```python
from build123d import *

# Parameters (mm, degrees)
EXTRUDE1_DEPTH                  = 75
F_1_2_0_500000_DIAMETER_HOLE1_D = 12.7
M6X1_0_TAPPED_HOLE1_D           = 6
LPATTERN1_COUNT                 = 2
LPATTERN1_PITCH                 = 25
LPATTERN1_COUNT_DIR2            = 2
LPATTERN1_PITCH_DIR2            = 25
M6X1_0_TAPPED_HOLE2_D           = 6
MIRROR2_COPY_1_D                = 6
MIRROR2_COPY_2_D                = 6
MIRROR2_COPY_3_D                = 6
MIRROR2_COPY_4_D                = 6
MIRROR3_COPY_1_D                = 6
MIRROR3_COPY_2_D                = 6
MIRROR3_COPY_3_D                = 6
MIRROR3_COPY_4_D                = 6
MIRROR3_COPY_5_D                = 6
MIRROR3_COPY_6_D                = 6
MIRROR3_COPY_7_D                = 6
MIRROR3_COPY_8_D                = 6
MIRROR3_COPY_9_D                = 6
MIRROR3_COPY_10_D               = 6


with BuildPart() as part:
    # Sketch1 → Extrude1 (new, symmetric)
    with BuildSketch(Plane.XY):
        Polygon((-67.79, 0), (67.79, 0), (67.79, 12.446), (75, 12.446), (75, 13.716), (-75, 13.716), (-75, 12.446), (-67.79, 12.446), align=None)
    extrude(amount=EXTRUDE1_DEPTH, both=True)

    # 1/2 (0.500000) Diameter Hole1 (through all)
    with Locations(Plane(origin=(0, 13.716, 0), x_dir=(-1, 0, 0), z_dir=(0, 1, 0))):
        with Locations((37.5, 25), (-37.5, 25), (-37.5, -25), (37.5, -25)):
            Hole(F_1_2_0_500000_DIAMETER_HOLE1_D / 2)

    # M6x1.0 Tapped Hole1 (through all)
    with Locations(Plane(origin=(0, 13.716, 0), x_dir=(-1, 0, 0), z_dir=(0, 1, 0))):
        with Locations((0, 0)):
            m6x1_0_tapped_hole1 = Hole(M6X1_0_TAPPED_HOLE1_D / 2)

    # LPattern1: M6x1.0 Tapped Hole1 2 × 2
    with Locations(*[(-i * LPATTERN1_PITCH, 0, -j * LPATTERN1_PITCH_DIR2) for i in range(LPATTERN1_COUNT) for j in range(LPATTERN1_COUNT_DIR2) if (i, j) != (0, 0)]):
        add(m6x1_0_tapped_hole1, mode=Mode.SUBTRACT)

    # M6x1.0 Tapped Hole2 (through all)
    with Locations(Plane(origin=(0, 13.716, 0), x_dir=(-1, 0, 0), z_dir=(0, 1, 0))):
        with Locations((37.5, -37.5), (50, -37.5), (50, -50)):
            m6x1_0_tapped_hole2 = Hole(M6X1_0_TAPPED_HOLE2_D / 2)

    # Mirror2: M6x1.0 Tapped Hole2 across plane
    add(m6x1_0_tapped_hole2.mirror(Plane.XY), mode=Mode.SUBTRACT)

    # Mirror2 copy 1 (through all)
    with Locations(Plane(origin=(0, 13.716, 25), x_dir=(-1, 0, 0), z_dir=(0, 1, 0))):
        with Locations((0, 0)):
            Hole(MIRROR2_COPY_1_D / 2)

    # Mirror2 copy 2 (through all)
    with Locations(Plane(origin=(-25, 13.716, 0), x_dir=(-1, 0, 0), z_dir=(0, 1, 0))):
        with Locations((0, 0)):
            Hole(MIRROR2_COPY_2_D / 2)

    # Mirror2 copy 3 (through all)
    with Locations(Plane(origin=(-25, 13.716, 25), x_dir=(-1, 0, 0), z_dir=(0, 1, 0))):
        with Locations((0, 0)):
            Hole(MIRROR2_COPY_3_D / 2)

    # Mirror2 copy 4 (through all)
    with Locations(Plane(origin=(0, 13.716, 0), x_dir=(-1, 0, 0), z_dir=(0, 1, 0))):
        with Locations((0, 0)):
            Hole(MIRROR2_COPY_4_D / 2)

    # Mirror3: M6x1.0 Tapped Hole2 across plane
    add(m6x1_0_tapped_hole2.mirror(Plane(origin=(0, 0, 0), x_dir=(0, 0, 1), z_dir=(1, 0, 0))), mode=Mode.SUBTRACT)

    # Mirror3 copy 1 (through all)
    with Locations(Plane(origin=(0, 13.716, -25), x_dir=(1, 0, 0), z_dir=(0, 1, 0))):
        with Locations((0, 0)):
            Hole(MIRROR3_COPY_1_D / 2)

    # Mirror3 copy 2 (through all)
    with Locations(Plane(origin=(25, 13.716, 0), x_dir=(1, 0, 0), z_dir=(0, 1, 0))):
        with Locations((0, 0)):
            Hole(MIRROR3_COPY_2_D / 2)

    # Mirror3 copy 3 (through all)
    with Locations(Plane(origin=(25, 13.716, -25), x_dir=(1, 0, 0), z_dir=(0, 1, 0))):
        with Locations((0, 0)):
            Hole(MIRROR3_COPY_3_D / 2)

    # Mirror3 copy 4 (through all)
    with Locations(Plane(origin=(0, 13.716, 0), x_dir=(1, 0, 0), z_dir=(0, 1, 0))):
        with Locations((0, 0)):
            Hole(MIRROR3_COPY_4_D / 2)

    # Mirror3 copy 5 (through all)
    with Locations(Plane(origin=(0, 13.716, 0), x_dir=(1, 0, 0), z_dir=(0, 1, 0))):
        with Locations((37.5, -37.5), (50, -37.5), (50, -50)):
            Hole(MIRROR3_COPY_5_D / 2)

    # Mirror3 copy 6 (through all)
    with Locations(Plane(origin=(0, 13.716, 25), x_dir=(1, 0, 0), z_dir=(0, 1, 0))):
        with Locations((0, 0)):
            Hole(MIRROR3_COPY_6_D / 2)

    # Mirror3 copy 7 (through all)
    with Locations(Plane(origin=(25, 13.716, 0), x_dir=(1, 0, 0), z_dir=(0, 1, 0))):
        with Locations((0, 0)):
            Hole(MIRROR3_COPY_7_D / 2)

    # Mirror3 copy 8 (through all)
    with Locations(Plane(origin=(25, 13.716, 25), x_dir=(1, 0, 0), z_dir=(0, 1, 0))):
        with Locations((0, 0)):
            Hole(MIRROR3_COPY_8_D / 2)

    # Mirror3 copy 9 (through all)
    with Locations(Plane(origin=(0, 13.716, 0), x_dir=(1, 0, 0), z_dir=(0, 1, 0))):
        with Locations((0, 0)):
            Hole(MIRROR3_COPY_9_D / 2)

    # Mirror3 copy 10 (through all)
    with Locations(Plane(origin=(0, 13.716, 0), x_dir=(1, 0, 0), z_dir=(0, 1, 0))):
        with Locations((0, 0)):
            Hole(MIRROR3_COPY_10_D / 2)


solid = part.part
```
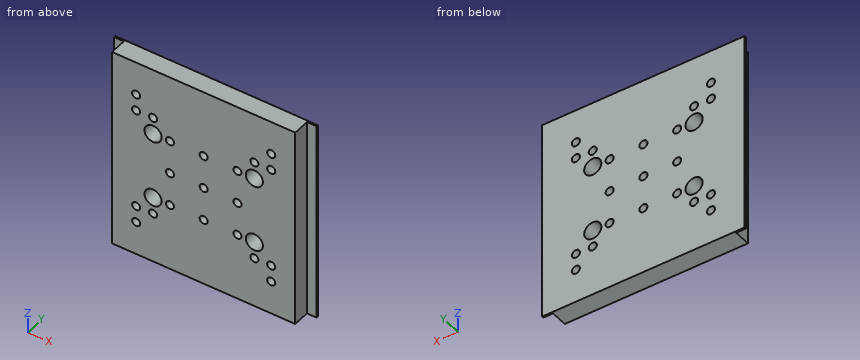
For this review, take the finished solid that the model builds, in its own axes (mm). Coordinates: 2 decimals unless noted, no trailing zeros. Order: outer loops, then holes, each group sorted by start corner. A loop starts at its lowest first (then second) coordinate and runs counter-clockwise, first axis right, second up. Notation, with made-up numbers: (-7.75, 18) - (22.25, 18) arc R27 ccw to (22.25, 36) - close; hole circle Ø7 at (-7, -36). An arc over 180 degrees is marked (long way). Answer as a JSON object with one key per item and string values. Group by question number.
1. We need section A-A on z = -25. State the section outline as (x, y) points.
2. For probe 1 along Z at (x, y) = (0, 5); probe 2 along Z at (x, y) = (37, 11); probe 3 along Z at (x, y) = (-39.5, 8), list the stretches that pass through material, from the lowest coordinate up.
3. Clearance check with flat-ended pins moving along their axes: P1, Ø3.5, axis at x = 0, z = -25, coming from the -Y side; P2, Ø3, axis at y = 9.5, z = -28, coming from the -X side. State where each tip first meets the part, or that it passes through.
4. We need section B-B on x = 37.5. State the section outline as (y, z) points, then the cut area to 3 significant figures.
5. We need section D-D on y = 5.25. Give the number of separate pieces and of enclosed holes in the cut face, then the cut area to 3 significant figures.
6. We need section C-C on z = 0. State the section outline as (x, y) points, then the cut area to 3 significant figures.
Final values:
{
 "1": {"outline": "(-75, 12.45) - (-67.79, 12.45) - (-67.79, 0) - (-43.85, 0) - (-43.85, 13.72) - (-75, 13.72) - close; (-31.15, 0) - (-28, 0) - (-28, 13.72) - (-31.15, 13.72) - close; (-22, 0) - (-3, 0) - (-3, 13.72) - (-22, 13.72) - close; (3, 0) - (22, 0) - (22, 13.72) - (3, 13.72) - close; (28, 0) - (31.15, 0) - (31.15, 13.72) - (28, 13.72) - close; (43.85, 0) - (67.79, 0) - (67.79, 12.45) - (75, 12.45) - (75, 13.72) - (43.85, 13.72) - close"},
 "2": {"probe 1": "-75 to -28, -22 to -3, 3 to 22, 28 to 75", "probe 2": "-75 to -40.46, -34.54 to -31.33, -18.67 to 18.67, 31.33 to 34.54, 40.46 to 75", "probe 3": "-75 to -39.74, -35.26 to -31.03, -18.97 to 18.97, 31.03 to 35.26, 39.74 to 75"},
 "3": {"P1": "through", "P2": "x = -67.79"},
 "4": {"outline": "(0, -75) - (13.72, -75) - (13.72, -40.5) - (0, -40.5) - close; (0, -34.5) - (13.72, -34.5) - (13.72, -31.35) - (0, -31.35) - close; (0, -18.65) - (13.72, -18.65) - (13.72, 18.65) - (0, 18.65) - close; (0, 31.35) - (13.72, 31.35) - (13.72, 34.5) - (0, 34.5) - close; (0, 40.5) - (13.72, 40.5) - (13.72, 75) - (0, 75) - close", "area": "1,540 mm²"},
 "5": {"separate pieces": "1", "enclosed holes": "25", "area": "19,200 mm²"},
 "6": {"outline": "(-75, 12.45) - (-67.79, 12.45) - (-67.79, 0) - (-28, 0) - (-28, 13.72) - (-75, 13.72) - close; (-22, 0) - (-3, 0) - (-3, 13.72) - (-22, 13.72) - close; (3, 0) - (22, 0) - (22, 13.72) - (3, 13.72) - close; (28, 0) - (67.79, 0) - (67.79, 12.45) - (75, 12.45) - (75, 13.72) - (28, 13.72) - close", "area": "1,630 mm²"}
}
